Could you check a few things on this model? Use its own coordinates, in mm. A direction names the side the tool comes from. Coordinates: 2 decimals unless noted, no trailing zeros. Write each loop counter-clockwise with the first axis right and the second up, starting at its lowest first coordinate (ties: lowest second). Pieces come first, ordered by that corner, then holes.
```python
from build123d import *

# Parameters (mm, degrees)
F0_W      = 62
F0_H      = 92
F1_DEPTH  = 2
F2_W      = 62
F2_H      = 92
F2_W_2    = 58
F2_H_2    = 88
F2_R      = 3
F3_DEPTH  = 28
F4_DEPTH  = 23
F5_R      = 1.25
F6_DEPTH  = 2
F7_R      = 1.25
F8_DEPTH  = 2
F9_R      = 1.25
F10_DEPTH = 2
F11_R     = 1.25
F12_DEPTH = 2
F14_DEPTH = 4
F15_R     = 1
F16_R     = 2
F17_R     = 4
F18_SIZE2 = 1
F18_SIZE  = 0.3639702343


with BuildPart() as f1:
    # F0 (on Top) → F1 (new body)
    with BuildSketch(Plane.XY):
        with Locations((31, 46)):
            Rectangle(F0_W, F0_H)
    extrude(amount=F1_DEPTH)

    # F2 (on face) → F3 (join)
    with BuildSketch(Plane.XY.offset(2)):
        with Locations((31, 46)):
            Rectangle(F2_W, F2_H)
        with Locations((31, 46)):
            Rectangle(F2_W_2, F2_H_2, mode=Mode.SUBTRACT)
        with Locations((7.5, 67)):
            Circle(F2_R)
        with Locations((56.5, 67)):
            Circle(F2_R)
        with Locations((7.5, 9)):
            Circle(F2_R)
        with Locations((56.5, 9)):
            Circle(F2_R)
    extrude(amount=F3_DEPTH)

    # F4 (cut): faces of the model
    f4_faces = [f1.faces().sort_by_distance(p)[0] for p in [
        (7.5, 67, 30),
        (56.5, 67, 30),
        (56.5, 9, 30),
        (7.5, 9, 30),
    ]]
    extrude(f4_faces, amount=-F4_DEPTH, mode=Mode.SUBTRACT)

    # F5 (on face) → F6 (join)
    with BuildSketch(Plane.XY.offset(7)):
        with Locations((7.5, 9)):
            Circle(F5_R)
    extrude(amount=F6_DEPTH)

    # F7 (on face) → F8 (join)
    with BuildSketch(Plane.XY.offset(7)):
        with Locations((56.5, 9)):
            Circle(F7_R)
    extrude(amount=F8_DEPTH)

    # F9 (on face) → F10 (join)
    with BuildSketch(Plane.XY.offset(7)):
        with Locations((56.5, 67)):
            Circle(F9_R)
    extrude(amount=F10_DEPTH)

    # F11 (on face) → F12 (join)
    with BuildSketch(Plane.XY.offset(7)):
        with Locations((7.5, 67)):
            Circle(F11_R)
    extrude(amount=F12_DEPTH)

    # F13 (on face) → F14 (cut)
    with BuildSketch(Plane.XZ):
        with BuildLine():
            ThreePointArc((38.5, 6), (38.2071067812, 6.7071067812), (37.5, 7))
            Line((37.5, 7), (26.5, 7))
            ThreePointArc((26.5, 7), (25.7928932188, 6.7071067812), (25.5, 6))
            Line((25.5, 6), (25.5, 0))
            Line((25.5, 0), (38.5, 0))
            Line((38.5, 0), (38.5, 6))
        make_face()
        with BuildLine():
            Line((48.5, 9.5), (47.5, 9.5))
            ThreePointArc((47.5, 9.5), (47.1464466094, 9.3535533906), (47, 9))
            ThreePointArc((47, 9), (47.1464466094, 8.6464466094), (47.5, 8.5))
            Line((47.5, 8.5), (48.5, 8.5))
            ThreePointArc((48.5, 8.5), (48.8535533906, 8.6464466094), (49, 9))
            ThreePointArc((49, 9), (48.8535533906, 9.3535533906), (48.5, 9.5))
        make_face()
        with BuildLine():
            Line((52.5, 9.5), (51.5, 9.5))
            ThreePointArc((51.5, 9.5), (51.1464466094, 9.3535533906), (51, 9))
            ThreePointArc((51, 9), (51.1464466094, 8.6464466094), (51.5, 8.5))
            Line((51.5, 8.5), (52.5, 8.5))
            ThreePointArc((52.5, 8.5), (52.8535533906, 8.6464466094), (53, 9))
            ThreePointArc((53, 9), (52.8535533906, 9.3535533906), (52.5, 9.5))
        make_face()
    extrude(amount=-F14_DEPTH, mode=Mode.SUBTRACT)

    # F15
    f15_edges = [f1.edges().sort_by_distance(p)[0] for p in [
        (25.5, 4, 1),
        (38.5, 4, 1),
    ]]
    fillet(f15_edges, radius=F15_R)

    # F16
    f16_edges = [f1.edges().sort_by_distance(p)[0] for p in [
        (2, 90, 16),
        (60, 90, 16),
        (60, 2, 16),
        (2, 2, 16),
    ]]
    fillet(f16_edges, radius=F16_R)

    # F17
    f17_edges = [f1.edges().sort_by_distance(p)[0] for p in [
        (0, 92, 15),
        (62, 92, 15),
        (62, 0, 15),
        (0, 0, 15),
    ]]
    fillet(f17_edges, radius=F17_R)

    # F18
    f18_edges = [f1.edges().sort_by_distance(p)[0] for p in [
        (51, 2, 9),
        (47, 2, 9),
    ]]
    f18_side = f1.faces().sort_by_distance((30.90829, 2, 16.53228))[0]
    chamfer(f18_edges, length=F18_SIZE, length2=F18_SIZE2, reference=f18_side)


solid = f1.part
```
1. On a 3-axis mill with a long thin cutter (end or side, diameter ignored), from which of +Z, -Z, +X, -X, +Y, -Y can I reach the whole of each face in a straight line? I mean faces 5 (the face through (31, 47, 0)), 6 (the face through (31, 47, 2)), 7 (the face through (32, 1, 7)). Say none if no direction works.
Verdict:
face 5: -Z, +X, -X, +Y, -Y
face 6: +Z
face 7: -Z, -Y
2. For pin 1 (3.5 mm diameter, centred on y = 1, z = 3.5, fed in from +X); pin 2 (3.5 mm diameter, centred on y = 1.5, z = 2, fed in from -X); pin 3 (3 mm diameter, centred on x = 56, y = 10, fed in from +Z), each with a flat end and sliding along its axis, tell me the tip position at first contact or that it passes through.
Verdict:
pin 1: stops at x = 61.8
pin 2: stops at x = 0.07
pin 3: stops at z = 9
3. I want a section at C-C on x = 7.5. Please give me the cut outline in (y, z), plus the area to 3 significant figures.
Verdict:
outline: (0, 0) - (92, 0) - (92, 30) - (90, 30) - (90, 2) - (70, 2) - (70, 7) - (68.25, 7) - (68.25, 9) - (65.75, 9) - (65.75, 7) - (64, 7) - (64, 2) - (12, 2) - (12, 7) - (10.25, 7) - (10.25, 9) - (7.75, 9) - (7.75, 7) - (6, 7) - (6, 2) - (2, 2) - (2, 30) - (0, 30) - close
area: 366 mm2
4. I want a section at A-A on z = 11. Please give me the cut outline in (x, y).
Verdict:
outline: (0, 4) arc R4 ccw to (4, 0) - (58, 0) arc R4 ccw to (62, 4) - (62, 88) arc R4 ccw to (58, 92) - (4, 92) arc R4 ccw to (0, 88) - close; hole (2, 4) arc R2 ccw to (4, 2) - (58, 2) arc R2 ccw to (60, 4) - (60, 88) arc R2 ccw to (58, 90) - (4, 90) arc R2 ccw to (2, 88) - close
5. I want a section at B-B on y = 9. Please give me the cut outline in (x, z).
Verdict:
outline: (0, 0) - (62, 0) - (62, 30) - (60, 30) - (60, 2) - (59.5, 2) - (59.5, 7) - (57.75, 7) - (57.75, 9) - (55.25, 9) - (55.25, 7) - (53.5, 7) - (53.5, 2) - (10.5, 2) - (10.5, 7) - (8.75, 7) - (8.75, 9) - (6.25, 9) - (6.25, 7) - (4.5, 7) - (4.5, 2) - (2, 2) - (2, 30) - (0, 30) - close
6. If we mould it in two halves opening along X, with no side actions, what happens to faces 1 (the face through (31, 0, 15)), 2 (the face through (60.797, 1.141, 15.21)), 3 (the face through (1.141, 90.797, 14.79)), 4 (the face through (57.172, 68.054, 7.986))? For each: pulls with the +X half, pulls with the -X half, needs draft (parallel to the pull), parting line crosses it, or undercut.
Verdict:
face 1: needs draft
face 2: pulls with the +X half
face 3: pulls with the -X half
face 4: undercut
7. Please list where these lines run through material, in increasing order: line 1 along X through (y, z) = (81.5, 26.5); line 2 along Y through (x, z) = (24, 14); line 3 along Z through (x, y) = (41, 65).
Verdict:
line 1: x = 0 to 2, 60 to 62
line 2: y = 0 to 2, 90 to 92
line 3: z = 0 to 2
8. I want a section at D-D on x = 15. Please give me the cut outline in (y, z).
Verdict:
outline: (0, 0) - (92, 0) - (92, 30) - (90, 30) - (90, 2) - (2, 2) - (2, 30) - (0, 30) - close
